Verification items for the finished model (mm, model axes). A direction names the side the tool comes from. Coordinates: 2 decimals unless noted, no trailing zeros. Order: outer loops, then holes, each group sorted by start corner. A loop starts at its lowest first (then second) coordinate and runs counter-clockwise, first axis right, second up. Notation, with made-up numbers: (6.25, 32.25) -> (46.25, 32.25) arc R10 cw to (46.25, 37.25) -> close; hole circle Ø4 at (5, 39.25). An arc over 180 degrees is marked (long way). Write each question's results on one line, items separated by ' | '. Start each with the question number.
(1) Go/stop test with flat-tipped pins: pin 1 (3 mm diameter, centred on x = -27.5, z = 5.5, fed in from -Y); pin 2 (8 mm diameter, centred on x = 27, z = 16.5, fed in from -Y); pin 3 (3 mm diameter, centred on x = -38, z = 5.5, fed in from +Y); pin 4 (12 mm diameter, centred on x = 68.5, z = 7, fed in from -Y). Record where each tip stops, or that it passes through.
(2) Set-up check for faces 1 (the cylindrical face through (88.193, 15.457, 17.395)), 2 (the cylindrical face through (97.15, -26.99, 5.07)), 3 (the flat face through (-30, 7.5, 5)), 4 (the flat face through (-32, -7.5, 5)): record each of +Z, -Z, +X, -X, +Y, -Y from which the full face is reachable in a straight line by a thin tool's end or side.
(3) Thickness scan on probe 1 along Y at (x, z) = (21, 2.5); probe 2 along Z at (x, y) = (45.5, -3); probe 3 along X at (y, z) = (-26, 1.5). Record the ranges inside material, lowest first. Write a range as [from, to].
(4) Draft check along Y on faces 5 (the flat face through (89, -10, 25)), 6 (the cylindrical face through (83.85, -10.28, 17.4)), 7 (the cylindrical face through (96.99, 27.15, 5.07)), 8 (the flat face through (61.733, -18.635, 4.93)). Enter one of: +Y half, -Y half, draft (parallel to the pull), parting line (faces both ways), or undercut.
(5) Cross-section at C-C on x = 10.5. Enter the section's corners in (y, z).
(6) Cross-section at B-B on y = -3.5. Enter the section's corners in (x, z), and give its area (3 significant figures).
(7) Cross-section at A-A on z = 13.75. Enter the section's corners in (x, y).
```python
from build123d import *

# Parameters (mm, degrees)
F0_R     = 5
F1_DEPTH = 10
F2_DEPTH = 25
F3_DEPTH = 25
F4_R     = 10
F5_R     = 20


with BuildPart() as f1:
    # F0 (on Top) → F1 (new body)
    with BuildSketch(Plane.XY):
        Polygon((80, 30), (43.835908, 7.5), (-100, 7.5), (-100, -7.5), (43.835908, -7.5), (80, -30), (100, -30), (100, 0), (100, 30), align=None)
        with Locations((88.843614, -10.5)):
            Circle(F0_R, mode=Mode.SUBTRACT)
        with Locations((88.843614, 10.5)):
            Circle(F0_R, mode=Mode.SUBTRACT)
        with Locations((88.843614, -10.5)):
            Circle(F0_R)
        with Locations((88.843614, 10.5)):
            Circle(F0_R)
    extrude(amount=F1_DEPTH)

    # F0 (on Top) → F2 (join)
    with BuildSketch(Plane.XY):
        with Locations((88.843614, -10.5)):
            Circle(F0_R)
    extrude(amount=F2_DEPTH)

    # F0 (on Top) → F3 (join)
    with BuildSketch(Plane.XY):
        with Locations((88.843614, 10.5)):
            Circle(F0_R)
    extrude(amount=F3_DEPTH)

    # F4
    f4_edges = [f1.edges().sort_by_distance(p)[0] for p in [
        (100, 30, 5),
        (100, -30, 5),
    ]]
    fillet(f4_edges, radius=F4_R)

    # F5
    f5_edges = [f1.edges().sort_by_distance(p)[0] for p in [
        (80, -30, 5),
        (80, 30, 5),
        (43.835908, 7.5, 5),
        (43.835908, -7.5, 5),
    ]]
    fillet(f5_edges, radius=F5_R)


solid = f1.part
```
Results are:
1) pin 1: stops at y = -7.5 | pin 2: passes through | pin 3: stops at y = 7.5 | pin 4: stops at y = -26.58
2) face 1: +Z | face 2: +Z, -Z, +X, -Y | face 3: +Z, -Z, -X, +Y | face 4: +Z, -Z, -X, -Y
3) probe 1: y = [-7.5, 7.5] | probe 2: z = [0, 10] | probe 3: x = [73.57, 98]
4) face 5: draft | face 6: undercut | face 7: +Y half | face 8: -Y half
5) outline: (-7.5, 0) -> (7.5, 0) -> (7.5, 10) -> (-7.5, 10) -> close
6) outline: (-100, 0) -> (100, 0) -> (100, 10) -> (-100, 10) -> close | area: 2,000 mm2
7) outline: circle Ø10 at (88.84, -10.5); circle Ø10 at (88.84, 10.5)
